Check sheet for the modelled part. Datum: model origin and axes. Units: mm. Round coordinates to 2 decimals unless told otherwise and drop trailing zeros. Order: outer loops, then holes, each group sorted by start corner. A loop starts at its lowest first (then second) coordinate and runs counter-clockwise, first axis right, second up. Notation, with made-up numbers: (31.25, 30.5) -> (77.25, 30.5) arc R11 ccw to (77.25, 35.5) -> close; hole circle Ø9 at (83, 26.25). An arc over 180 degrees is marked (long way). Answer in a Markdown table with one row per item.
from build123d import *

# Parameters (mm, degrees)
SKETCH1_R           = 6.257840103
BOSS_EXTRUDE1_DEPTH = 3
SKETCH2_R           = 8.121320344
CUT_EXTRUDE1_DEPTH  = 10.344577331


with BuildPart() as part:
    # Sketch1 → Boss-Extrude1 (new body)
    with BuildSketch(Plane(origin=(0, 0, 0), x_dir=(1, 0, 0), z_dir=(0, 1, 0))):
        with Locations(Location((0, 0, 0), (0, 0, 270))):
            Circle(SKETCH1_R)
    extrude(amount=BOSS_EXTRUDE1_DEPTH)

    # Sketch2 → Cut-Extrude1 (cut, through all)
    with BuildSketch(Plane(origin=(0, 3, 0), x_dir=(1, 0, 0), z_dir=(0, 1, 0))):
        Circle(SKETCH2_R)
        Polygon((6.121320344, -2.535533906), (6.121320344, 2.535533906), (2.535533906, 6.121320344), (-2.535533906, 6.121320344), (-6.121320344, 2.535533906), (-6.121320344, -2.535533906), (-2.535533906, -6.121320344), (2.535533906, -6.121320344), align=None, mode=Mode.SUBTRACT)
    extrude(amount=-CUT_EXTRUDE1_DEPTH, mode=Mode.SUBTRACT)


solid = part.part
Item 1: Cross-section at A-A (y = 0.2). Record the boundary of the cut face in (x, z), and give its area (3 significant figures).
Result sheet:
| item | result |
|---|---|
| outline | (-6.12, -1.3) arc R6.26 ccw to (-5.25, -3.41) -> (-3.41, -5.25) arc R6.26 ccw to (-1.3, -6.12) -> (1.3, -6.12) arc R6.26 ccw to (3.41, -5.25) -> (5.25, -3.41) arc R6.26 ccw to (6.12, -1.3) -> (6.12, 1.3) arc R6.26 ccw to (5.25, 3.41) -> (3.41, 5.25) arc R6.26 ccw to (1.3, 6.12) -> (-1.3, 6.12) arc R6.26 ccw to (-3.41, 5.25) -> (-5.25, 3.41) arc R6.26 ccw to (-6.12, 1.3) -> close |
| area | 121 mm^2 |
Item 2: Cross-section at C-C (x = 5.5). Record the boundary of the cut face in (y, z).
Result sheet:
| item | result |
|---|---|
| outline | (0, -2.99) -> (3, -2.99) -> (3, 2.99) -> (0, 2.99) -> close |
Item 3: Depth check by flat-ended pin: P1, Ø1, axis at x = -3, y = 2.5, coming from the -Z side. Enter the tip coordinate at first touch or a pass-through.
Result sheet:
| item | result |
|---|---|
| P1 | stops at z = -5.74 |
Item 4: Cross-section at B-B (z = 2.75). Record the boundary of the cut face in (x, y).
Result sheet:
| item | result |
|---|---|
| outline | (-5.62, 0) -> (5.62, 0) -> (5.62, 3) -> (-5.62, 3) -> close |
Item 5: Scan lines: line 1 (Z direction, x = 3, y = 1.6); line 2 (X direction, y = 0.75, z = 3.25); line 3 (Z direction, x = 4.5, y = 1.1). Record each from-to range of solid material in increasing order. Write a range as [from, to].
Result sheet:
| item | result |
|---|---|
| line 1 | z = [-5.49, 5.49] |
| line 2 | x = [-5.35, 5.35] |
| line 3 | z = [-4.16, 4.16] |
